Can you work these out from the model? Positions are in its coordinate system, mm. A direction names the side the tool comes from. Give positions to 0.01 mm unless a question says otherwise; leave off trailing zeros. Write each loop counter-clockwise with the first axis right and the second up, starting at its lowest first coordinate (ties: lowest second). Pieces come first, ordered by that corner, then holes.
from build123d import *

# Parameters (mm, degrees)
AXIAL_HOLES_DEPTH      = 184.274684558
AXIAL_HOLES_DEPTH_BACK = 184.274684558
SKETCH2_R              = 1.65


with BuildPart() as part:
    # Axial profile (mm) → Full revolution (revolve)
    with BuildSketch(Plane.XY, mode=Mode.PRIVATE) as full_revolution_sk:
        Polygon((169.7, 25.6), (174.7, 25.6), (174.7, 24), (176.7, 24), (176.7, 34.4), (169.7, 34.4), align=None)
    revolve(full_revolution_sk.sketch.rotate(Axis((-110, 0, 0), (1, 0, 0)), 90), axis=Axis((-110, 0, 0), (1, 0, 0)))

    # Sketch2 → Axial holes (cut, two sides: drawn at the far end of the back side and taken through both)
    with BuildSketch(Plane(origin=(0, 0, 0), x_dir=(0, 0, -1), z_dir=(1, 0, 0)).offset(-AXIAL_HOLES_DEPTH_BACK)):
        with Locations(Location((29.4, 0, 0), (0, 0, 180))):
            Circle(SKETCH2_R)
        with Locations(Location((-14.7, 25.461146871, 0), (0, 0, 180))):
            Circle(SKETCH2_R)
        with Locations(Location((-14.7, -25.461146871, 0), (0, 0, 180))):
            Circle(SKETCH2_R)
    extrude(amount=AXIAL_HOLES_DEPTH + AXIAL_HOLES_DEPTH_BACK, mode=Mode.SUBTRACT)


solid = part.part
(1) Imagine slicing it at B-B, the plane z = 0. Write out the boundary of the cut face in (x, y).
Returned:
outline: (169.7, -34.4) - (176.7, -34.4) - (176.7, -24) - (174.7, -24) - (174.7, -25.6) - (169.7, -25.6) - close; (169.7, 25.6) - (174.7, 25.6) - (174.7, 24) - (176.7, 24) - (176.7, 34.4) - (169.7, 34.4) - close
(2) Imagine slicing it at A-A, the plane y = 0. Write out the boundary of the cut face in (x, z).
Returned:
outline: (169.7, -34.4) - (176.7, -34.4) - (176.7, -31.05) - (169.7, -31.05) - close; (169.7, -27.75) - (176.7, -27.75) - (176.7, -24) - (174.7, -24) - (174.7, -25.6) - (169.7, -25.6) - close; (169.7, 25.6) - (174.7, 25.6) - (174.7, 24) - (176.7, 24) - (176.7, 34.4) - (169.7, 34.4) - close
(3) If I drill on L1, parallel to Y at x = 173.75, z = 0.5; L2, parallel to Y at x = 176.15, z = 0; L3, parallel to Z at x = 171.5, y = -2, over which ranges is the centre line in solid material (lowest first)?
Returned:
L1: y = -34.4 to -25.6, 25.6 to 34.4
L2: y = -34.4 to -24, 24 to 34.4
L3: z = -34.34 to -25.52, 25.52 to 34.34
(4) If we mould it in two halves opening along Z, with no side actions, what happens to faces 1 (the face through (173.151, -1.513, -34.367)), 2 (the face through (173.15, -26.85, 15.59)), 3 (the face through (169.7, -26, 0))? For each: +Z half, -Z half, draft (parallel to the pull), parting line (faces both ways), or undercut.
Returned:
face 1: parting line
face 2: undercut
face 3: draft
(5) For faces 4 (the face through (175.71, -7.21, 22.89)), 5 (the face through (174.7, -23, -8)), which set-ups out of +Z, -Z, +X, -X, +Y, -Y let a thin tool reach every point of the face, with its end or its side?
Returned:
face 4: +X, -X
face 5: -X
(6) Imagine slicing it at C-C, the plane y = -13.5. Write out the boundary of the cut face in (x, z).
Returned:
outline: (169.7, -31.64) - (176.7, -31.64) - (176.7, -19.84) - (174.7, -19.84) - (174.7, -21.75) - (169.7, -21.75) - close; (169.7, 21.75) - (174.7, 21.75) - (174.7, 19.84) - (176.7, 19.84) - (176.7, 31.64) - (169.7, 31.64) - close
(7) Will these pins go through, and if not, where does the flat tip stop? P1, Ø2, axis at x = 170.5, z = 20, coming from the -Y side; P2, Ø2.5, axis at y = 25.46, z = 14.7, coming from the -X side; P3, Ø4, axis at x = 175.5, z = 8.5, coming from the +Y side; P4, Ø2, axis at x = 170.5, y = -19.5, coming from the -Z side.
Returned:
P1: stops at y = -28.68
P2: passes through
P3: stops at y = 33.78
P4: stops at z = -29
(8) Imagine slicing it at D-D, the plane z = 14.7. Write out the boundary of the cut face in (x, y).
Returned:
outline: (169.7, -31.1) - (176.7, -31.1) - (176.7, -27.11) - (169.7, -27.11) - close; (169.7, -23.81) - (176.7, -23.81) - (176.7, -18.97) - (174.7, -18.97) - (174.7, -20.96) - (169.7, -20.96) - close; (169.7, 20.96) - (174.7, 20.96) - (174.7, 18.97) - (176.7, 18.97) - (176.7, 23.81) - (169.7, 23.81) - close; (169.7, 27.11) - (176.7, 27.11) - (176.7, 31.1) - (169.7, 31.1) - close
